```python
from build123d import *

# Parameters (mm, degrees)
CHAMFER1_SIZE      = 0.3
CUT_EXTRUDE1_DEPTH = 1


with BuildPart() as part:
    # Sketch2 → Revolve2 (revolve)
    with BuildSketch(Plane.XY, mode=Mode.PRIVATE) as revolve2_sk:
        with BuildLine():
            Line((18.5, 0), (-18.5, 0))
            Line((-18.5, 0), (-20.15, 0))
            Line((-20.15, 0), (-20.15, 1.43))
            ThreePointArc((-20.15, 1.43), (-19.604204204, 2.235398215), (-18.85, 2.85))
            Line((-18.85, 2.85), (-18.5, 2.85))
            Line((-18.5, 2.85), (-18.5, 1.5))
            Line((-18.5, 1.5), (18.5, 1.5))
            Line((18.5, 1.5), (18.5, 0))
        make_face()
    revolve(revolve2_sk.sketch.rotate(Axis((18.5, 0, 0), (-1, 0, 0)), 90), axis=Axis((18.5, 0, 0), (-1, 0, 0)))

    # Chamfer1
    chamfer1_edges = [part.edges().sort_by_distance(p)[0] for p in [
        (18.5, 0, 1.5),
    ]]
    chamfer(chamfer1_edges, length=CHAMFER1_SIZE)

    # Sketch3 → Cut-Extrude1 (cut)
    with BuildSketch(Plane.ZY.offset(20.15)):
        Polygon((-1, 0.577350269), (-1, -0.577350269), (0, -1.154700538), (1, -0.577350269), (1, 0.577350269), (0, 1.154700538), align=None)
    extrude(amount=-CUT_EXTRUDE1_DEPTH, mode=Mode.SUBTRACT)


solid = part.part
```
The listing builds one solid part. Answer for the finished solid, in the listing's coordinates (mm). A direction names the side the tool comes from. Coordinates: 2 decimals unless noted, no trailing zeros. Write each loop counter-clockwise with the first axis right and the second up, starting at its lowest first coordinate (ties: lowest second). Pieces come first, ordered by that corner, then holes.
Q1. Section A-A, the plane x = 13.5 is taken. Write down the section's boundary in (y, z).
Returned:
outline: circle Ø3 at (0, 0)
Q2. Which of the six approach directions +Z, -Z, +X, -X, +Y, -Y give full straight-line access (tool end or side, diameter ignored) to faces 1 (the flat face through (18.5, 0, 0)), 2 (the flat face through (-19.7, 0, -1))?
Returned:
face 1: +Z, -Z, +X, +Y, -Y
face 2: -X
Q3. Find the intervals of material crossed by line 1 along X through (y, z) = (-0.1, 0.7); line 2 along Y through (x, z) = (2, -0.15), in increasing order.
Returned:
line 1: x = -19.15 to 18.5
line 2: y = -1.49 to 1.49
Q4. The mould has two halves that part along Y. Classify faces 3 (the flat face through (-18.5, 1.2, -1.2)), 4 (the cylindrical face through (0.11, -0.45, -1.43)), 5 (the flat face through (-19.66, 0.87, -0.49)): released by +Y, released by -Y, zero draft, split by the parting line, or undercut.
Returned:
face 3: zero draft
face 4: split by the parting line
face 5: undercut
Q5. Given P1, Ø1.5, axis at x = -3, y = 0, coming from the -Z side; P2, Ø2, axis at x = 2, z = -2, coming from the +Y side; P3, Ø1.1, axis at x = -20, y = 0, coming from the -Z side, each flat-ended and moving along its own axis, determine where each tip first touches the part or whether it passes through.
Returned:
P1: stops at z = -1.5
P2: stops at y = 1.12
P3: stops at z = -2.39
